from build123d import *

# Parameters (mm, degrees)
BOSS_EXTRUDE1_DEPTH   = 5
BOSS_EXTRUDE2_DEPTH   = 20
FILLET1_R             = 5
F_3_0MM_DOWEL_HOLE1_D = 3


with BuildPart() as part:
    # Sketch1 → Boss-Extrude1 (new body)
    with BuildSketch(Plane.XY):
        Polygon((-47.026906911, 0), (32.973093089, 1.057571587), (31.842813456, 86.557571587), (-48.157186544, 85.5), align=None)
    extrude(amount=BOSS_EXTRUDE1_DEPTH)

    # Sketch2 → Boss-Extrude2 (add)
    with BuildSketch(Plane.XY):
        Polygon((-33.681834279, 85.691359016), (-33.681834279, 80.691359016), (-13.681834279, 80.691359016), (-13.681834279, 85.955751912), align=None)
        Polygon((11.908900131, 86.294052332), (11.908900131, 81.558445229), (31.908900131, 81.558445229), (31.908900131, 86.558445229), align=None)
        Polygon((-37.027780592, 0.132184899), (-37.027780592, 5.132184899), (-17.027780592, 5.132184899), (-17.027780592, 0.396577795), align=None)
        Polygon((12.907006414, 0.792305048), (12.907006414, 6.056697944), (32.907006414, 6.056697944), (32.907006414, 1.056697944), align=None)
    extrude(amount=BOSS_EXTRUDE2_DEPTH)

    # Fillet1
    fillet1_edges = [part.edges().sort_by_distance(p)[0] for p in [
        (-33.681834279, 83.191359016, 20),
        (-13.681834279, 83.323555464, 20),
        (31.908900131, 84.058445229, 20),
        (11.908900131, 83.926248781, 20),
        (-17.027780592, 2.764381347, 20),
        (-37.027780592, 2.632184899, 20),
        (32.907006414, 3.556697944, 20),
        (12.907006414, 3.424501496, 20),
    ]]
    fillet(fillet1_edges, radius=FILLET1_R)

    # Ø3.0mm Dowel Hole1 (through all)
    with Locations(Plane(origin=(-1.138496573, 86.121570382, 0), x_dir=(0.9999126319463549, 0.013218489857520067, 0), z_dir=(-0.013218489857520067, 0.9999126319463549, 0))):
        with Locations((-22.546181203, -15), (23.048536729, -15)):
            Hole(F_3_0MM_DOWEL_HOLE1_D / 2)


solid = part.part
The model under review builds one solid part; all positions refer to its coordinate system, in mm. A direction names the side the tool comes from. Give positions to 0.01 mm unless a question says otherwise; leave off trailing zeros. Loops run counter-clockwise (first coordinate to the right, second up) from the corner with the lowest first, then second, coordinate; pieces in that order, holes last. Notation, with made-up numbers: (-13.5, 70) -> (26.5, 70) arc R20 cw to (26.5, 83) -> close; hole circle Ø11 at (66.25, 88). An arc over 180 degrees is marked (long way). Put each result on its own line as item: value. Start each with the question number.
1. For faces 1 (the face through (-27, 5.132, 12)), 2 (the face through (12.907, 3, 10)), list the 3-axis set-ups (+Z, -Z, +X, -X, +Y, -Y) from which the entire face can be reached by the end or side of a thin tool; tool diameter is ignored.
2. Clearance check with flat-ended pins moving along their axes: P1, Ø5.5, axis at y = 83, z = 8, coming from the -X side; P2, Ø3, axis at x = 9.5, y = 18, coming from the -Z side; P3, Ø1.4, axis at y = 3.5, z = 10.5, coming from the +X side; P4, Ø10, axis at x = -30.5, y = 48.5, coming from the +Z side. State where each tip first meets the part, or that it passes through.
3. Mouldability with a two-part tool opening along Y and no side actions: class faces 3 (the face through (-33.682, 83, 10)), 4 (the face through (-24, 80.691, 12)) as released by +Y, released by -Y, zero draft, split by the parting line, or undercut.
4. We need section B-B on x = -16. State the section outline as (y, z) points, then the cut area to 3 significant figures.
5. We need section A-A on z = 7.5. State the section outline as (x, y) points.
6. We need section C-C on y = 13. State the section outline as (x, z) points, then the cut area to 3 significant figures.
7. Wall thickness on probe 1 along Z at (x, y) = (6, 33.5); probe 2 along Y at (x, z) = (23, 6.5); probe 3 along Y at (x, z) = (-25, 12): over which ranges is each line inside the solid? List them lowest first.
Determined:
1. face 1: +Z, -X
1. face 2: +Z, -Y
2. P1: x = -33.68
2. P2: z = 0
2. P3: x = 32.91
2. P4: z = 5
3. face 3: zero draft
3. face 4: undercut
4. outline: (0.41, 0) -> (85.93, 0) -> (85.93, 19.22) -> (80.69, 19.22) -> (80.69, 5) -> (0.41, 5) -> close
4. area: 502 mm^2
5. outline: (-37.03, 0.13) -> (-17.03, 0.4) -> (-17.03, 5.13) -> (-37.03, 5.13) -> close; (-33.68, 80.69) -> (-13.68, 80.69) -> (-13.68, 85.96) -> (-33.68, 85.69) -> close; (11.91, 81.56) -> (31.91, 81.56) -> (31.91, 86.56) -> (11.91, 86.29) -> close; (12.91, 0.79) -> (32.91, 1.06) -> (32.91, 6.06) -> (12.91, 6.06) -> close
6. outline: (-47.2, 0) -> (32.82, 0) -> (32.82, 5) -> (-47.2, 5) -> close
6. area: 400 mm^2
7. probe 1: 0 to 5
7. probe 2: 0.93 to 6.06, 81.56 to 86.44
7. probe 3: 0.29 to 5.13, 80.69 to 85.81
